from build123d import *

# Parameters (mm, degrees)
SKETCH_1_W          = 40
SKETCH_1_H          = 43
SKETCH_1_R          = 1.5
EXTRUDE_1_DEPTH     = 6
CUT_EXTRUDE_1_DEPTH = 46.806658905
SKETCH_3_R          = 13
EXTRUDE_2_DEPTH     = 4
SKETCH_4_R          = 13
SKETCH_4_R_2        = 12.2
EXTRUDE_3_DEPTH     = 5
SKETCH_5_R          = 3.5
CUT_EXTRUDE_2_DEPTH = 33.973474188


with BuildPart() as part:
    # 草图1 → 凸台-拉伸1 (new body)
    with BuildSketch(Plane.XY):
        Rectangle(SKETCH_1_W, SKETCH_1_H)
        Circle(SKETCH_1_R, mode=Mode.SUBTRACT)
    extrude(amount=EXTRUDE_1_DEPTH)

    # 草图2 → 切除-拉伸1 (cut, through all)
    with BuildSketch(Plane(origin=(20, 0, 0), x_dir=(0, 0, -1), z_dir=(1, 0, 0))):
        with BuildLine():
            ThreePointArc((-2, 16.5), (-2.292893219, 17.207106781), (-3, 17.5))
            Line((-3, 17.5), (-3, 15.5))
            ThreePointArc((-3, 15.5), (-2.292893219, 15.792893219), (-2, 16.5))
        make_face()
        with BuildLine():
            Line((-3, 15.5), (-3, 17.5))
            ThreePointArc((-3, 17.5), (-4, 16.5), (-3, 15.5))
        make_face()
        with BuildLine():
            ThreePointArc((-2, -16.5), (-2.292893219, -15.792893219), (-3, -15.5))
            Line((-3, -15.5), (-3, -17.5))
            ThreePointArc((-3, -17.5), (-2.292893219, -17.207106781), (-2, -16.5))
        make_face()
        with BuildLine():
            Line((-3, -17.5), (-3, -15.5))
            ThreePointArc((-3, -15.5), (-4, -16.5), (-3, -17.5))
        make_face()
    extrude(amount=-CUT_EXTRUDE_1_DEPTH, mode=Mode.SUBTRACT)

    # 草图3 → 凸台-拉伸2 (add)
    with BuildSketch(Plane(origin=(0, 0, 0), x_dir=(-1, 0, 0), z_dir=(0, 0, -1))):
        Circle(SKETCH_3_R)
    extrude(amount=EXTRUDE_2_DEPTH)

    # 草图4 → 凸台-拉伸3 (add)
    with BuildSketch(Plane(origin=(0, 0, -4), x_dir=(-1, 0, 0), z_dir=(0, 0, -1))):
        Circle(SKETCH_4_R)
        Circle(SKETCH_4_R_2, mode=Mode.SUBTRACT)
    extrude(amount=EXTRUDE_3_DEPTH)

    # 草图5 → 切除-拉伸2 (cut, through all)
    with BuildSketch(Plane.XY.offset(6)):
        Circle(SKETCH_5_R)
    extrude(amount=-CUT_EXTRUDE_2_DEPTH, mode=Mode.SUBTRACT)


solid = part.part
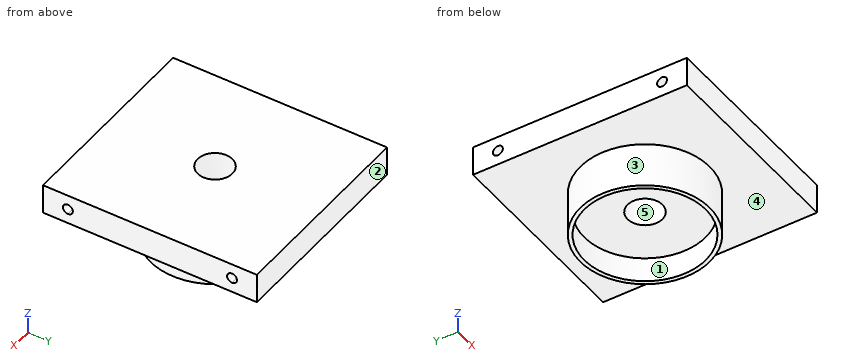
Design review of the part built by this model. Coordinates are the model's own, in mm. Face numbers are marked on the shaded views. A direction names the side the tool comes from. Give positions to 0.01 mm unless a question says otherwise; leave off trailing zeros. Write each loop counter-clockwise with the first axis right and the second up, starting at its lowest first coordinate (ties: lowest second). Pieces come first, ordered by that corner, then holes. Notation, with made-up numbers: M 46,31.5 L 98,31.5 A13 ccw 98,48.5 Z; hole C 10.25,75 d6. An arc over 180 degrees is marked long. Return JSON: item names as keys, results as strings. Group by question number.
Item 1: The part is to be moulded in two halves that separate along X. For the marked faces 3, 4 and 5, say which applies: pulls with the +X half, pulls with the -X half, needs draft (parallel to the pull), parting line crosses it, or undercut.
Item 2: Take a section at D-D (x = 15). Give the boundary of the cut face in (y, z).
Item 3: Take a section at A-A (x = 0). Give the boundary of the cut face in (y, z).
Item 4: Tool access review of the marked faces 1 and 2: name each direction out of +Z, -Z, +X, -X, +Y, -Y from which nothing blocks a thin tool from reaching the whole face with its end or side.
Item 5: Take a section at B-B (y = 0). Give the boundary of the cut face in (x, z), plus the area to 3 significant figures.
Item 6: Clearance check with flat-ended pins moving along their axes: pin 1 Ø12 at (x, y) = (5, -5) entering from -Z; pin 2 Ø4 at (x, y) = (0, 0) entering from +Z; pin 3 Ø1 at (x, y) = (12.5, 9) entering from -Z; pin 4 Ø2 at (x, z) = (-3.5, -3) entering from +Y. State where each tip first meets the part, or that it passes through.
Item 7: Take a section at C-C (z = 0.5). Give the boundary of the cut face in (x, y), plus the area to 3 significant figures.
Item 8: Wall thickness on line 1 along Y through (x, z) = (0, -1.25); line 2 along Y through (x, z) = (2, 3.75); line 3 along Z through (x, y) = (14, 16.5): over which ranges is each line inside the solid? List them lowest first.
Return value:
{
 "1": {"face 3": "parting line crosses it", "face 4": "needs draft", "face 5": "undercut"},
 "2": {"outline": "M -21.5,0 L 21.5,0 L 21.5,6 L -21.5,6 Z; hole C -16.5,3 d2; hole C 16.5,3 d2"},
 "3": {"outline": "M -21.5,0 L -13,0 L -13,-9 L -12.2,-9 L -12.2,-4 L -3.5,-4 L -3.5,6 L -21.5,6 Z; M 3.5,-4 L 12.2,-4 L 12.2,-9 L 13,-9 L 13,0 L 21.5,0 L 21.5,6 L 3.5,6 Z; hole C -16.5,3 d2; hole C 16.5,3 d2"},
 "4": {"face 1": "-Z", "face 2": "+Z, -Z, +X, -X, +Y"},
 "5": {"outline": "M -20,0 L -13,0 L -13,-9 L -12.2,-9 L -12.2,-4 L -3.5,-4 L -3.5,6 L -20,6 Z; M 3.5,-4 L 12.2,-4 L 12.2,-9 L 13,-9 L 13,0 L 20,0 L 20,6 L 3.5,6 Z", "area": "282 mm2"},
 "6": {"pin 1": "stops at z = -9", "pin 2": "passes through", "pin 3": "stops at z = 0", "pin 4": "stops at y = 12.76"},
 "7": {"outline": "M -20,-21.5 L 20,-21.5 L 20,21.5 L -20,21.5 Z; hole C 0,0 d7", "area": "1,680 mm2"},
 "8": {"line 1": "y = -13 to -3.5, 3.5 to 13", "line 2": "y = -21.5 to -17.16, -15.84 to -2.87, 2.87 to 15.84, 17.16 to 21.5", "line 3": "z = 0 to 2, 4 to 6"}
}
